```python
from build123d import *

# Parameters (mm, degrees)
BOSS_EXTRUDE1_DEPTH = 70.5
SKETCH2_R           = 1.5
BOSS_EXTRUDE2_DEPTH = 5


with BuildPart() as part:
    # Sketch1 → Boss-Extrude1 (new, symmetric)
    with BuildSketch(Plane(origin=(0, 0, 0), x_dir=(0, 0, -1), z_dir=(1, 0, 0))):
        Polygon((0, 0), (133.046623313, -35.649735272), (136.43225101, -33.451082938), (0, 3.105828541), align=None)
    extrude(amount=BOSS_EXTRUDE1_DEPTH, both=True)

    # Sketch2 → Boss-Extrude2 (add)
    with BuildSketch(Plane.ZY.offset(66.5)):
        Polygon((0, 0), (0, -24.852850374), (-49.318516526, -24.852850374), (-49.318516526, -13.214856675), align=None)
        with Locations((-20, -14.676469472)):
            Circle(SKETCH2_R, mode=Mode.SUBTRACT)
        with Locations((-39.318516526, -19.852850374)):
            Circle(SKETCH2_R, mode=Mode.SUBTRACT)
    boss_extrude2 = extrude(amount=-BOSS_EXTRUDE2_DEPTH)

    # Mirror1: Boss-Extrude2 across plane
    add(boss_extrude2.mirror(Plane(origin=(0, 0, 0), x_dir=(0, 0, 1), z_dir=(1, 0, 0))))


solid = part.part
```
Geometry check sheet. Reference: the model listing, model coordinates, mm. A direction names the side the tool comes from. Round coordinates to 2 decimals unless told otherwise and drop trailing zeros. Order: outer loops, then holes, each group sorted by start corner. A loop starts at its lowest first (then second) coordinate and runs counter-clockwise, first axis right, second up. Notation, with made-up numbers: (24, 5.25) - (46, 5.25) arc R22 cw to (46, 39.25) - close; hole circle Ø8 at (58.5, 80.5). An arc over 180 degrees is marked (long way). Use a Markdown table: item, result. Add a question column.
(1) Sectioned sample at C-C, the plane y = -28.5. Enter the section's corners in (x, z), and give its area (3 significant figures).
(2) Depth check by flat-ended pin: pin 1 (6 mm diameter, centred on y = -19.5, z = -71.5, fed in from +X); pin 2 (5 mm diameter, centred on x = 23, z = -41.5, fed in from -Y); pin 3 (6 mm diameter, centred on x = 55, z = -46.5, fed in from +Y); pin 4 (1 mm diameter, centred on x = -34, z = -39, fed in from -Y). Enter the tip coordinate at first touch or a pass-through.
(3) Material ranges on line 1 along X through (y, z) = (-10, -27); line 2 along Y through (x, z) = (-63.9, -20); line 3 along Y through (x, z) = (19, -44.5), recorded low to high. Write a range as [from, to].
(4) Sectioned sample at B-B, the plane x = -36. Enter the section's corners in (y, z), and give its area (3 significant figures).
(5) Release check for a two-part mould opening along Y. For faces 6 (the flat face through (70.5, -16, -68)), 7 (the cylindrical face through (64.035, -20.766, -40.509)), 8 (the flat face through (0.99, -15.43, -69.17)) record: pulls with the +Y half, pulls with the -Y half, needs draft (parallel to the pull), parting line crosses it, or undercut.
(6) Tool access check on faces 1 (the flat face through (64, -19, -49.319)), 2 (the flat face through (64, -24.853, -24)), 3 (the flat face through (-66.5, -15, -24)), 4 (the flat face through (61.5, -15, -24)), 5 (the flat face through (66.5, -15, -24)). Record the directions out of +Z, -Z, +X, -X, +Y, -Y that give a thin tool (end or side, any length) a straight path to the whole face; none if there is none.
(7) Sectioned sample at A-A, the plane z = -46. Enter the section's corners in (x, y).
Answers below:
| question | item | result |
|---|---|---|
| 1 | outline | (-70.5, -117.95) - (70.5, -117.95) - (70.5, -106.36) - (-70.5, -106.36) - close |
| 1 | area | 1,630 mm² |
| 2 | pin 1 | x = 70.5 |
| 2 | pin 2 | y = -11.79 |
| 2 | pin 3 | y = -8.55 |
| 2 | pin 4 | y = -10.58 |
| 3 | line 1 | [-66.5, -61.5], [61.5, 66.5] |
| 3 | line 2 | [-24.85, -16.18], [-13.18, -2.25] |
| 3 | line 3 | [-11.92, -8.82] |
| 4 | outline | (-35.65, -133.05) - (-33.45, -136.43) - (3.11, 0) - (0, 0) - close |
| 4 | area | 418 mm² |
| 5 | face 6 | needs draft |
| 5 | face 7 | undercut |
| 5 | face 8 | pulls with the +Y half |
| 6 | face 1 | +X, -X, -Y |
| 6 | face 2 | +Z, +X, -X, -Y |
| 6 | face 3 | +Z, -X, -Y |
| 6 | face 4 | +Z, -Y |
| 6 | face 5 | +Z, +X, -Y |
| 7 | outline | (-70.5, -12.33) - (-66.5, -12.33) - (-66.5, -24.85) - (-61.5, -24.85) - (-61.5, -12.33) - (61.5, -12.33) - (61.5, -24.85) - (66.5, -24.85) - (66.5, -12.33) - (70.5, -12.33) - (70.5, -9.22) - (-70.5, -9.22) - close |
